Could you check a few things on this model? Use its own coordinates, in mm. Round coordinates to 2 decimals unless told otherwise and drop trailing zeros. Write each loop counter-clockwise with the first axis right and the second up, starting at its lowest first coordinate (ties: lowest second). Pieces come first, ordered by that corner, then holes. Notation, with made-up numbers: (-21, -12) -> (31, -12) arc R31 cw to (31, 26) -> close; hole circle Ø2 at (-5, 68.25). An arc over 180 degrees is marked (long way). One line per question, with ' | ' between items. Start each with the question number.
1. If I drill on line 1 along X through (y, z) = (2.2, 0); line 2 along Z through (x, y) = (13.5, 3.05); line 3 along X through (y, z) = (1.7, 0.5), over which ranges is the centre line in solid material (lowest first)? Write a range as [from, to].
2. For pin 1 Ø3 at (x, y) = (20.5, 3) entering from -Z; pin 2 Ø3 at (y, z) = (3, 4) entering from -X; pin 3 Ø1.5 at (x, y) = (-22.5, 2.5) entering from -Z, each with a flat end and sliding along its axis, tell me the tip position at first contact or that it passes through.
3. Imagine slicing it at D-D, the plane x = 21.5. List the corners of the cut face in (y, z) for me.
4. Imagine slicing it at A-A, the plane x = -16. List the corners of the cut face in (y, z) for me.
5. Imagine slicing it at B-B, the plane y = 1.55. List the corners of the cut face in (x, z) for me, and give its area (3 significant figures).
6. Imagine slicing it at C-C, the plane z = -13. List the corners of the cut face in (x, y) for me.
from build123d import *

# Parameters (mm, degrees)
BOSS_EXTRUDE1_DEPTH = 5
SKETCH2_R           = 1.75
SKETCH2_W           = 5
SKETCH2_H           = 5
CUT_EXTRUDE1_DEPTH  = 5
CHAMFER1_SIZE       = 1


with BuildPart() as part:
    # Sketch1 → Boss-Extrude1 (new body)
    with BuildSketch(Plane(origin=(0, 0, 0), x_dir=(1, 0, 0), z_dir=(0, 1, 0))):
        Polygon((-28.867513459, 0), (-14.43375673, -25), (14.43375673, -25), (28.867513459, 0), (14.43375673, 25), (-14.43375673, 25), align=None)
    extrude(amount=BOSS_EXTRUDE1_DEPTH)

    # Sketch2 → Cut-Extrude1 (cut)
    with BuildSketch(Plane(origin=(0, 5, 0), x_dir=(1, 0, 0), z_dir=(0, 1, 0))):
        with Locations(Location((-23.867513459, 0, 0), (0, 0, 270))):
            Circle(SKETCH2_R)
        with Locations(Location((23.867513459, 0, 0), (0, 0, 270))):
            Circle(SKETCH2_R)
        with Locations((-14.137513459, 0)):
            Rectangle(SKETCH2_W, SKETCH2_H)
        with Locations((14.137513459, 0)):
            Rectangle(SKETCH2_W, SKETCH2_H)
    extrude(amount=-CUT_EXTRUDE1_DEPTH, mode=Mode.SUBTRACT)

    # Chamfer1
    chamfer1_edges = [part.edges().sort_by_distance(p)[0] for p in [
        (-11.637513459, 5, 0),
        (-14.137513459, 5, -2.5),
        (-16.637513459, 5, 0),
        (-14.137513459, 5, 2.5),
        (16.637513459, 5, 0),
        (14.137513459, 5, -2.5),
        (11.637513459, 5, 0),
        (14.137513459, 5, 2.5),
    ]]
    chamfer(chamfer1_edges, length=CHAMFER1_SIZE)


solid = part.part
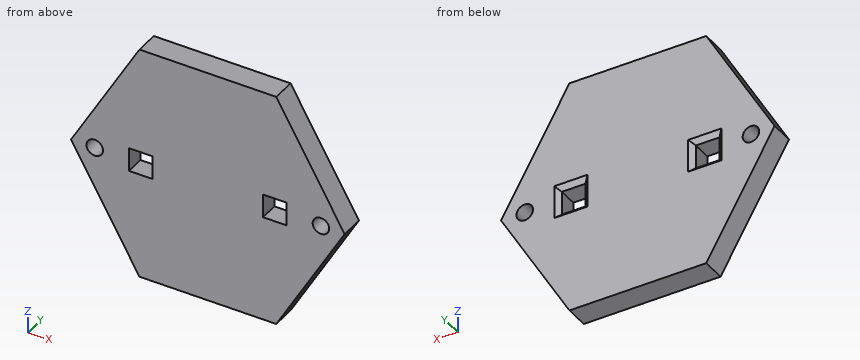
Geometry results:
1) line 1: x = [-28.87, -25.62], [-22.12, -16.64], [-11.64, 11.64], [16.64, 22.12], [25.62, 28.87] | line 2: z = [-25, -2.5], [2.5, 25] | line 3: x = [-28.58, -25.54], [-22.19, -16.64], [-11.64, 11.64], [16.64, 22.19], [25.54, 28.58]
2) pin 1: stops at z = -17.09 | pin 2: stops at x = -27.42 | pin 3: stops at z = -12.33
3) outline: (0, -12.76) -> (5, -12.76) -> (5, 12.76) -> (0, 12.76) -> close
4) outline: (0, -22.29) -> (5, -22.29) -> (5, -3.5) -> (4, -2.5) -> (0, -2.5) -> close; (0, 2.5) -> (4, 2.5) -> (5, 3.5) -> (5, 22.29) -> (0, 22.29) -> close
5) outline: (-28.87, 0) -> (-14.43, -25) -> (14.43, -25) -> (28.87, 0) -> (14.43, 25) -> (-14.43, 25) -> close; hole circle Ø3.5 at (-23.87, 0); hole (-16.64, -2.5) -> (-11.64, -2.5) -> (-11.64, 2.5) -> (-16.64, 2.5) -> close; hole (11.64, -2.5) -> (16.64, -2.5) -> (16.64, 2.5) -> (11.64, 2.5) -> close; hole circle Ø3.5 at (23.87, 0) | area: 2,100 mm2
6) outline: (-21.36, 0) -> (21.36, 0) -> (21.36, 5) -> (-21.36, 5) -> close
